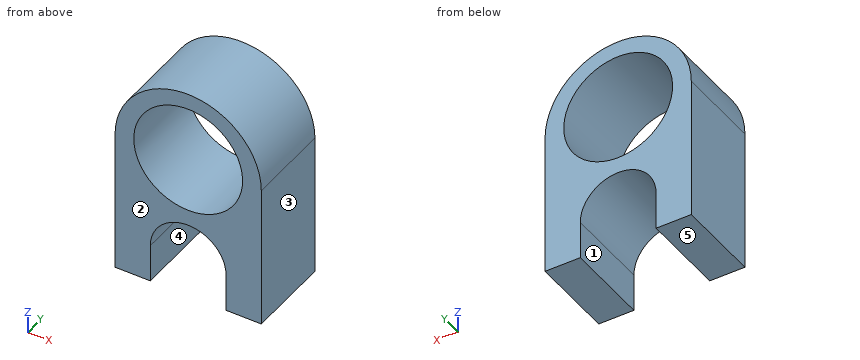
```python
from build123d import *

# Parameters (mm, degrees)
SZKIC1_W                    = 54
SZKIC1_H                    = 31.5
DODANIE_WYCI_GNI_CIE1_DEPTH = 45
SZKIC2_W                    = 54
SZKIC2_H                    = 31.5
DODANIE_WYCI_GNI_CIE2_DEPTH = 35
WYTNIJ_WYCI_GNI_CIE3_REACH  = 63.207
ZAOKR_GLENIE1_RADIUS        = 27
ZAOKR_GLENIE1_LENGTH        = 31.5
SZKIC9_R                    = 20.1
WYTNIJ_WYCI_GNI_CIE4_DEPTH  = 62.206617289


with BuildPart() as part:
    # Szkic1 → Dodanie-wyciągnięcie1 (new body)
    with BuildSketch(Plane.XY):
        Rectangle(SZKIC1_W, SZKIC1_H)
    extrude(amount=DODANIE_WYCI_GNI_CIE1_DEPTH)

    # Szkic2 → Dodanie-wyciągnięcie2 (add)
    with BuildSketch(Plane(origin=(0, 0, 0), x_dir=(-1, 0, 0), z_dir=(0, 0, -1))):
        Rectangle(SZKIC2_W, SZKIC2_H)
    extrude(amount=DODANIE_WYCI_GNI_CIE2_DEPTH)

    # Szkic8 → Wytnij-wyciągnięcie3 (cut, up to next)
    with BuildSketch(Plane(origin=(0, 15.75, 0), x_dir=(1, 0, 0), z_dir=(0, 1, 0)), mode=Mode.PRIVATE) as wytnij_wyci_gni_cie3_sk1:
        with BuildLine():
            Line((14, 35), (-14, 35))
            Line((-14, 35), (-14, 21))
            ThreePointArc((-14, 21), (0, 7), (14, 21))
            Line((14, 21), (14, 35))
        make_face()
    wytnij_wyci_gni_cie3_tool1 = extrude(wytnij_wyci_gni_cie3_sk1.sketch, amount=-WYTNIJ_WYCI_GNI_CIE3_REACH, mode=Mode.PRIVATE) & part.part
    add(wytnij_wyci_gni_cie3_tool1.solids().sort_by_distance((0, 15.75, -22.306898))[0], mode=Mode.SUBTRACT)

    # Zaokrąglenie1: full round fillet: the end face becomes a half cylinder, R = half its width
    zaokr_glenie1_face = Plane((0, 0, 45), x_dir=(0, -1, 0), z_dir=(0, 0, 1))  # on the end face: x along it, z out of the body
    zaokr_glenie1_slab = zaokr_glenie1_face.offset(-ZAOKR_GLENIE1_RADIUS / 2) * Box(ZAOKR_GLENIE1_LENGTH, 2 * ZAOKR_GLENIE1_RADIUS, ZAOKR_GLENIE1_RADIUS, mode=Mode.PRIVATE)  # the body's end, R deep
    zaokr_glenie1_round = Plane((0, 0, 18), x_dir=(0, 0, 1), z_dir=(0, -1, 0)) * Cylinder(ZAOKR_GLENIE1_RADIUS, ZAOKR_GLENIE1_LENGTH, mode=Mode.PRIVATE)  # its axis R under the face
    add(zaokr_glenie1_slab - zaokr_glenie1_round, mode=Mode.SUBTRACT)

    # Szkic9 → Wytnij-wyciągnięcie4 (cut, through all)
    with BuildSketch(Plane(origin=(0, -15.75, 0), x_dir=(-1, 0, 0), z_dir=(0, -1, 0))):
        with Locations(Location((0, -19, 0), (0, 0, 90))):
            Circle(SZKIC9_R)
    extrude(amount=-WYTNIJ_WYCI_GNI_CIE4_DEPTH, mode=Mode.SUBTRACT)


solid = part.part
```
Check sheet for the modelled part. Datum: model origin and axes. Units: mm. Face numbers are marked on the shaded views. A direction names the side the tool comes from. Coordinates: 2 decimals unless noted, no trailing zeros. Loops run counter-clockwise (first coordinate to the right, second up) from the corner with the lowest first, then second, coordinate; pieces in that order, holes last. Notation, with made-up numbers: M 57.25,14.5 L 84.25,14.5 A32 cw 84.25,46.5 Z; hole C 62,-30.5 d6. An arc over 180 degrees is marked long. Answer as a JSON object with one key per item and string values.
1. Scan lines: L1, parallel to X at y = -1.5, z = 19; L2, parallel to Z at x = -0.5, y = -6.5; L3, parallel to X at y = -8, z = -31. Record each from-to range of solid material in increasing order. Write a range as from..to.
Outcome:
{"L1": "-26.98..-20.1, 20.1..26.98", "L2": "-7.01..-1.09, 39.09..45", "L3": "-27..-14, 14..27"}
2. Depth check by flat-ended pin: P1, Ø6, axis at x = 14, y = -6.5, coming from the +Z side; P2, Ø10, axis at x = 3.5, y = 0, coming from the -Z side; P3, Ø2, axis at x = -8.5, y = -12, coming from the -Z side. Enter the tip coordinate at first touch or a pass-through.
Outcome:
{"P1": "z = 42.66", "P2": "z = -9.88", "P3": "z = -10.72"}
3. Access from +Z, -Z, +X, -X, +Y, -Y to the whole of each face (thin tool, end or side, straight path). Record for the marked faces 4 and 5.
Outcome:
{"face 4": "-Z, +Y, -Y", "face 5": "-Z, +X, -X, +Y, -Y"}
4. Sectioned sample at C-C on z = 16.5. Record the cut outline in (x, y).
Outcome:
{"outline": "M -27,-15.75 L -19.94,-15.75 L -19.94,15.75 L -27,15.75 Z; M 19.94,-15.75 L 27,-15.75 L 27,15.75 L 19.94,15.75 Z"}
5. Sectioned sample at D-D on x = 22. Record the cut outline in (y, z), and give its area (3 significant figures).
Outcome:
{"outline": "M -15.75,-35 L 15.75,-35 L 15.75,33.65 L -15.75,33.65 Z", "area": "2,160 mm²"}
6. Release check for a two-part mould opening along X. For the marked faces 1, 2 and 3 record: pulls with the +X half, pulls with the -X half, needs draft (parallel to the pull), parting line crosses it, or undercut.
Outcome:
{"face 1": "undercut", "face 2": "needs draft", "face 3": "pulls with the +X half"}
7. Sectioned sample at B-B on y = 4. Record the cut outline in (x, z), and give its area (3 significant figures).
Outcome:
{"outline": "M -27,-35 L -14,-35 L -14,-21 A14 cw 14,-21 L 14,-35 L 27,-35 L 27,18 A27 ccw -27,18 Z; hole C 0,19 d40.2", "area": "2,040 mm²"}
8. Sectioned sample at A-A on x = 0. Record the cut outline in (y, z), and give its area (3 significant figures).
Outcome:
{"outline": "M -15.75,-7 L 15.75,-7 L 15.75,-1.1 L -15.75,-1.1 Z; M -15.75,39.1 L 15.75,39.1 L 15.75,45 L -15.75,45 Z", "area": "372 mm²"}
